CAD build for the part. Positions are in the model's coordinates, mm. Face numbers are marked on the shaded views. A direction names the side the tool comes from. Round coordinates to 2 decimals unless told otherwise and drop trailing zeros. Order: outer loops, then holes, each group sorted by start corner. A loop starts at its lowest first (then second) coordinate and runs counter-clockwise, first axis right, second up. Notation, with made-up numbers: (15, 21) - (54, 21) arc R23 ccw to (54, 33) - close; hole circle Ø8 at (26, 64). An arc over 180 degrees is marked (long way). Use one line per item in the form item = value. Start each with the question number.
from build123d import *

# Parameters (mm, degrees)
SKETCH_1_W          = 22.3
SKETCH_1_H          = 17
EXTRUDE_1_DEPTH     = 1.5
SKETCH_2_W          = 6
SKETCH_2_H          = 6
SKETCH_2_W_2        = 5
SKETCH_2_H_2        = 2.5
SKETCH_2_W_3        = 2
SKETCH_2_H_3        = 4
EXTRUDE_2_DEPTH     = 2.7
SKETCH_3_R          = 0.75
CUT_EXTRUDE_1_DEPTH = 15.278042583


with BuildPart() as part:
    # 스케치1 → 보스-돌출1 (new body)
    with BuildSketch(Plane(origin=(0, 0, 0), x_dir=(1, 0, 0), z_dir=(0, 1, 0))):
        Rectangle(SKETCH_1_W, SKETCH_1_H)
    extrude(amount=EXTRUDE_1_DEPTH)

    # 스케치2 → 보스-돌출2 (add)
    with BuildSketch(Plane(origin=(0, 1.5, 0), x_dir=(1, 0, 0), z_dir=(0, 1, 0))):
        with Locations((4.55, 3.5)):
            Rectangle(SKETCH_2_W, SKETCH_2_H)
        with Locations((-4.65, 6.75)):
            Rectangle(SKETCH_2_W_2, SKETCH_2_H_2)
        with Locations((-8.95, 0)):
            Rectangle(SKETCH_2_W_3, SKETCH_2_H_3)
        with Locations((8.95, 0)):
            Rectangle(SKETCH_2_W_3, SKETCH_2_H_3)
        with Locations((-2.45, -0.5)):
            Rectangle(SKETCH_2_W_2, SKETCH_2_H_3)
    extrude(amount=EXTRUDE_2_DEPTH)

    # 스케치3 → 컷-돌출1 (cut, through all)
    with BuildSketch(Plane(origin=(0, 1.5, 0), x_dir=(1, 0, 0), z_dir=(0, 1, 0))):
        with Locations((-11.15, 7)):
            Circle(SKETCH_3_R)
        with Locations((-11.15, 4)):
            Circle(SKETCH_3_R)
        with Locations(Location((-9.15, 7, 0), (0, 0, 270))):
            Circle(SKETCH_3_R)
        with Locations(Location((-9.15, 4, 0), (0, 0, 270))):
            Circle(SKETCH_3_R)
        with Locations(Location((9.15, 7, 0), (0, 0, 270))):
            Circle(SKETCH_3_R)
        with Locations((11.15, 7)):
            Circle(SKETCH_3_R)
        with Locations(Location((9.15, 4, 0), (0, 0, 270))):
            Circle(SKETCH_3_R)
        with Locations((11.15, 4)):
            Circle(SKETCH_3_R)
        with Locations((-11.15, -4)):
            Circle(SKETCH_3_R)
        with Locations(Location((-9.15, -4, 0), (0, 0, 270))):
            Circle(SKETCH_3_R)
        with Locations(Location((-9.15, -7, 0), (0, 0, 270))):
            Circle(SKETCH_3_R)
        with Locations((-11.15, -7)):
            Circle(SKETCH_3_R)
        with Locations((11.15, -4)):
            Circle(SKETCH_3_R)
        with Locations(Location((9.15, -4, 0), (0, 0, 270))):
            Circle(SKETCH_3_R)
        with Locations(Location((9.15, -7, 0), (0, 0, 270))):
            Circle(SKETCH_3_R)
        with Locations((11.15, -7)):
            Circle(SKETCH_3_R)
    extrude(amount=-CUT_EXTRUDE_1_DEPTH, mode=Mode.SUBTRACT)


solid = part.part
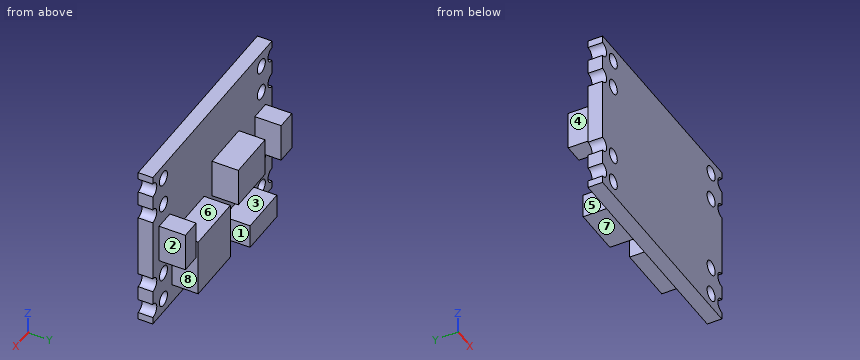
(1) Flat gauge pins, fed straight in: P1, Ø1.4, axis at y = 2.5, z = 0, coming from the +X side; P2, Ø1, axis at x = 8.5, y = 3, coming from the -Z side; P3, Ø1, axis at x = 7, z = 5, coming from the +Y side; P4, Ø0.9, axis at x = -9.15, z = 4, coming from the +Y side. Where does each tip first touch, or does it go through?
(2) Slice it at D-D (y = 3.3). Give the cut face in (x, z), and give its area (3 significant figures).
(3) Which spindle directions (+Z, -Z, +X, -X, +Y, -Y) get a long thin tool onto all of the face, cutting with end or side? Do the marked faces 5, 6, 7 and 8. Say none if no direction does.
(4) Slice it at B-B (y = 1.05). Give the number of separate pieces and of enclosed holes in the cut face, and give its area (3 significant figures).
(5) Slice it at C-C (x = -9.15). Give the cut face in (y, z), and give its area (3 significant figures).
(6) Mould opens along X. For the marked faces 1, 2, 3 and 4 say: pulls with the +X half, pulls with the -X half, needs draft (parallel to the pull), parting line crosses it, or undercut.
(7) Slice it at A-A (z = -7). Give the cut face in (x, y).
(8) Wall check: line 1 (X direction, y = 0.5, z = -7); line 2 (Y direction, x = -5, z = -3); line 3 (X direction, y = 1.6, z = -3.5). Give the ranges that are in metal, low to high. Write a range as [from, to].
Results list:
q1.P1 = 9.95
q1.P2 = -2
q1.P3 = 1.5
q1.P4 = through
q2.outline = (-9.95, -2) - (-7.95, -2) - (-7.95, 2) - (-9.95, 2) - close; (-7.15, -8) - (-2.15, -8) - (-2.15, -5.5) - (-7.15, -5.5) - close; (-4.95, -1.5) - (0.05, -1.5) - (0.05, 2.5) - (-4.95, 2.5) - close; (1.55, -6.5) - (7.55, -6.5) - (7.55, -0.5) - (1.55, -0.5) - close; (7.95, -2) - (9.95, -2) - (9.95, 2) - (7.95, 2) - close
q2.area = 84.5 mm²
q3.face_5 = +Z, -Z, -X, +Y
q3.face_6 = +Z, +Y
q3.face_7 = -Z, +X, -X, +Y
q3.face_8 = +Z, -Z, +Y
q4.separate_pieces = 1
q4.enclosed_holes = 8
q4.area = 358 mm²
q5.outline = (0, -8.5) - (1.5, -8.5) - (1.5, -7.75) - (0, -7.75) - close; (0, -6.25) - (1.5, -6.25) - (1.5, -4.75) - (0, -4.75) - close; (0, -3.25) - (1.5, -3.25) - (1.5, -2) - (4.2, -2) - (4.2, 2) - (1.5, 2) - (1.5, 3.25) - (0, 3.25) - close; (0, 4.75) - (1.5, 4.75) - (1.5, 6.25) - (0, 6.25) - close; (0, 7.75) - (1.5, 7.75) - (1.5, 8.5) - (0, 8.5) - close
q5.area = 27.3 mm²
q6.face_1 = undercut
q6.face_2 = pulls with the +X half
q6.face_3 = needs draft
q6.face_4 = pulls with the -X half
q7.outline = (-10.4, 0) - (-9.9, 0) - (-9.9, 1.5) - (-10.4, 1.5) - close; (-8.4, 0) - (8.4, 0) - (8.4, 1.5) - (-2.15, 1.5) - (-2.15, 4.2) - (-7.15, 4.2) - (-7.15, 1.5) - (-8.4, 1.5) - close; (9.9, 0) - (10.4, 0) - (10.4, 1.5) - (9.9, 1.5) - close
q8.line_1 = [-10.4, -9.9], [-8.4, 8.4], [9.9, 10.4]
q8.line_2 = [0, 1.5]
q8.line_3 = [1.55, 7.55]
